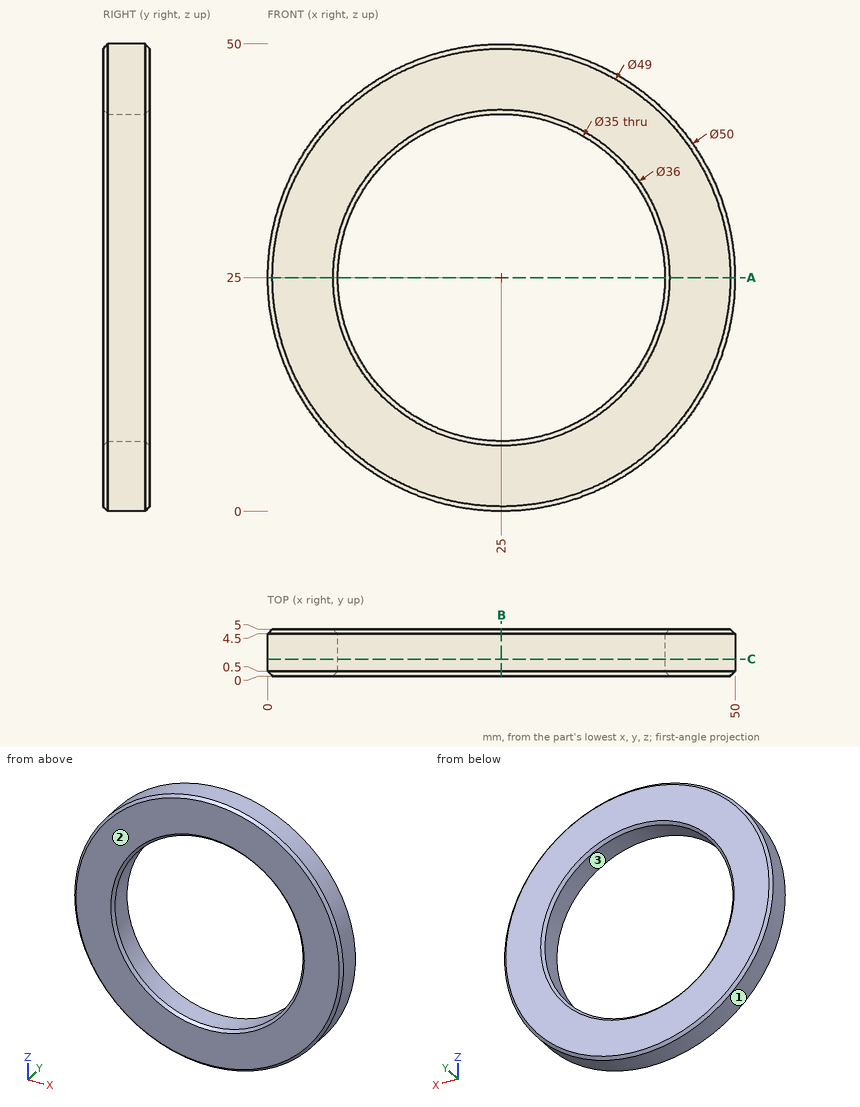
Check sheet for the drawn part. Datum: minimum x, y, z corner. Units: mm. Round coordinates to 2 decimals unless told otherwise and drop trailing zeros. Order: outer loops, then holes, each group sorted by start corner. A loop starts at its lowest first (then second) coordinate and runs counter-clockwise, first axis right, second up. Notation, with made-up numbers: M 82.5,8 L 117.5,8 A18 ccw 117.5,25 Z; hole C -7.75,51 d7. An arc over 180 degrees is marked long. Answer in a Markdown table with one row per item.
(1) Gauge pin test, flat ends, axial feed: pin 1 (8 mm diameter, centred on x = 15.5, z = 24.5, fed in from +Y); pin 2 (1 mm diameter, centred on y = 1, z = 32.5, fed in from -X). Record the tip position at first contact, or that the pin passes through.
Findings:
| item | result |
|---|---|
| pin 1 | passes through |
| pin 2 | stops at x = 1 |
(2) Section check A-A on z = 25. Record the boundary of the cut face in (x, y).
Findings:
| item | result |
|---|---|
| outline | M 0,0.5 L 0.5,0 L 7,0 L 7.5,0.5 L 7.5,4.5 L 7,5 L 0.5,5 L 0,4.5 Z; M 42.5,0.5 L 43,0 L 49.5,0 L 50,0.5 L 50,4.5 L 49.5,5 L 43,5 L 42.5,4.5 Z |
(3) Draft check along X on the marked faces 1, 2 and 3. Enter one of: +X half, -X half, draft (parallel to the pull), parting line (faces both ways), or undercut.
Findings:
| item | result |
|---|---|
| face 1 | parting line |
| face 2 | draft |
| face 3 | undercut |
(4) Section check B-B on x = 25. Record the boundary of the cut face in (y, z), plus the area to 3 significant figures.
Findings:
| item | result |
|---|---|
| outline | M 0,0.5 L 0.5,0 L 4.5,0 L 5,0.5 L 5,7 L 4.5,7.5 L 0.5,7.5 L 0,7 Z; M 0,43 L 0.5,42.5 L 4.5,42.5 L 5,43 L 5,49.5 L 4.5,50 L 0.5,50 L 0,49.5 Z |
| area | 74.0 mm^2 |
(5) Section check C-C on y = 1.8. Record the boundary of the cut face in (x, z), plus the area to 3 significant figures.
Findings:
| item | result |
|---|---|
| outline | C 25,25 d50; hole C 25,25 d35 |
| area | 1,000 mm^2 |
(6) Material ranges on line 1 along Z through (x, y) = (25, 2.9); line 2 along Z through (x, y) = (38.5, 1.6); line 3 along X through (y, z) = (0.95, 23), recorded low to high. Write a range as from..to.
Findings:
| item | result |
|---|---|
| line 1 | z = 0..7.5, 42.5..50 |
| line 2 | z = 3.96..13.86, 36.14..46.04 |
| line 3 | x = 0.08..7.61, 42.39..49.92 |
